Geometry: final body of the model. Coordinates: model frame, mm. Round coordinates to 2 decimals unless told otherwise and drop trailing zeros. Answer as a JSON object with one key per item and string values. Group by question number.
Item 1: Section A-A (y = 17). Count the separate pieces of the cut face and the enclosed holes in it, plus the area to 3 significant figures.
Item 2: First-contact query: pin 1 (4 mm diameter, centred on y = 19.5, z = 4, fed in from +X); pin 2 (1.2 mm diameter, centred on x = 67.5, z = -5, fed in from +Y). Flat tips, straight axial feed; report the tip coordinate or a pass-through.
Item 3: Line query: line 1 (X direction, y = 1, z = 27); line 2 (X direction, y = 2, z = -27); line 3 (Z direction, x = 100, y = 1.2). Output: solid intervals per line, ascending.
```python
from build123d import *

# Parameters (mm, degrees)
BOSS_EXTRUDE1_DEPTH  = 130
SKETCH2_R            = 3
CUT_EXTRUDE1_DEPTH   = 139.706225167
M3_CLEARANCE_HOLE1_D = 3.4


with BuildPart() as part:
    # Sketch1 → Boss-Extrude1 (new body)
    with BuildSketch(Plane(origin=(0, 0, 0), x_dir=(0, 0, -1), z_dir=(1, 0, 0))):
        Polygon((-40.13, 0), (-40.13, 30), (-39.48, 30), (-39.48, 3), (-37.068076923, 3), (-37.068076923, 30), (-36.418076923, 30), (-36.418076923, 3), (-34.006153846, 3), (-34.006153846, 30), (-33.356153846, 30), (-33.356153846, 3), (-30.944230769, 3), (-30.944230769, 30), (-30.294230769, 30), (-30.294230769, 3), (-27.882307692, 3), (-27.882307692, 30), (-27.232307692, 30), (-27.232307692, 3), (-24.820384615, 3), (-24.820384615, 30), (-24.170384615, 30), (-24.170384615, 3), (-21.758461538, 3), (-21.758461538, 30), (-21.108461538, 30), (-21.108461538, 3), (-18.696538462, 3), (-18.696538462, 30), (-18.046538462, 30), (-18.046538462, 3), (-15.634615385, 3), (-15.634615385, 30), (-14.984615385, 30), (-14.984615385, 3), (-12.572692308, 3), (-12.572692308, 30), (-11.922692308, 30), (-11.922692308, 3), (-9.510769231, 3), (-9.510769231, 30), (-8.860769231, 30), (-8.860769231, 3), (-6.448846154, 3), (-6.448846154, 30), (-5.798846154, 30), (-5.798846154, 3), (-3.386923077, 3), (-3.386923077, 30), (-2.736923077, 30), (-2.736923077, 3), (-0.325, 3), (-0.325, 30), (0.325, 30), (0.325, 3), (2.736923077, 3), (2.736923077, 30), (3.386923077, 30), (3.386923077, 3), (5.798846154, 3), (5.798846154, 30), (6.448846154, 30), (6.448846154, 3), (8.860769231, 3), (8.860769231, 30), (9.510769231, 30), (9.510769231, 3), (11.922692308, 3), (11.922692308, 30), (12.572692308, 30), (12.572692308, 3), (14.984615385, 3), (14.984615385, 30), (15.634615385, 30), (15.634615385, 3), (18.046538462, 3), (18.046538462, 30), (18.696538462, 30), (18.696538462, 3), (21.108461538, 3), (21.108461538, 30), (21.758461538, 30), (21.758461538, 3), (24.170384615, 3), (24.170384615, 30), (24.820384615, 30), (24.820384615, 3), (27.232307692, 3), (27.232307692, 30), (27.882307692, 30), (27.882307692, 3), (30.294230769, 3), (30.294230769, 30), (30.944230769, 30), (30.944230769, 3), (33.356153846, 3), (33.356153846, 30), (34.006153846, 30), (34.006153846, 3), (36.418076923, 3), (36.418076923, 30), (37.068076923, 30), (37.068076923, 3), (39.48, 3), (39.48, 30), (40.13, 30), (40.13, 3), (40.13, 0), align=None)
    extrude(amount=BOSS_EXTRUDE1_DEPTH)

    # Sketch2 → Cut-Extrude1 (cut, through all)
    with BuildSketch(Plane(origin=(0, 3, 0), x_dir=(1, 0, 0), z_dir=(0, 1, 0))):
        with Locations((10, 27)):
            Circle(SKETCH2_R)
        with Locations((100, 27)):
            Circle(SKETCH2_R)
        with Locations((65, 30.944230769)):
            Circle(SKETCH2_R)
        with Locations((10, -27)):
            Circle(SKETCH2_R)
        with Locations((55, -27)):
            Circle(SKETCH2_R)
        with Locations((100, -27)):
            Circle(SKETCH2_R)
    extrude(amount=CUT_EXTRUDE1_DEPTH, mode=Mode.SUBTRACT)

    # M3 Clearance Hole1 (through all)
    with Locations(Plane(origin=(10, 3, -27), x_dir=(0, 0, 1), z_dir=(0, 1, 0))):
        with Locations((0, 0), (-3.944230769, 55), (0, 90), (54, 0), (54, 45), (54, 90)):
            Hole(M3_CLEARANCE_HOLE1_D / 2)


solid = part.part
```
Values:
{
 "1": {"separate pieces": "38", "enclosed holes": "0", "area": "2,250 mm^2"},
 "2": {"pin 1": "stops at x = 130", "pin 2": "stops at y = 3"},
 "3": {"line 1": "x = 0 to 8.3, 11.7 to 53.3, 56.7 to 98.3, 101.7 to 130", "line 2": "x = 0 to 8.3, 11.7 to 98.3, 101.7 to 130", "line 3": "z = -40.13 to -28.7, -25.3 to 25.3, 28.7 to 40.13"}
}
